Input: part model. Units: mm. Frame: model coordinates. A direction names the side the tool comes from. Round coordinates to 2 decimals unless told otherwise and drop trailing zeros. Loops run counter-clockwise (first coordinate to the right, second up) from the corner with the lowest first, then second, coordinate; pieces in that order, holes last. Notation, with made-up numbers: M 12,78.5 L 34,78.5 A26 cw 34,96.5 Z; hole C 69.5,42.25 d3. An arc over 180 degrees is marked long. Return JSON: item names as keys, results as strings. Group by question number.
1) Access query for faces 1 (the face through (40, -1, 10)), 2 (the face through (-115, 95, 20)), 3 (the face through (-1, 1, 20)), 4 (the face through (-40, -1, 10)). Directions: +Z, -Z, +X, -X, +Y, -Y. A direction counts if a zero-diameter tool reaches every point of the face in a straight line with its end or side. Return the directions, or none.
2) Contact query for flat-ended pins moving along their axis: P1, Ø8, axis at y = -4, z = 23.5, coming from the -X side; P2, Ø8, axis at x = 3.5, y = -25.5, coming from the +Z side; P3, Ø20, axis at x = -53.5, z = 19.5, coming from the -Y side. Output: stop coordinate, or through.
3) Section D-D (x = -71.5). Output: boundary loops of the cut face in (y, z), plus the area to 3 significant figures.
4) Section B-B (x = -32). Output: boundary loops of the cut face in (y, z), plus the area to 3 significant figures.
5) Section A-A (z = 7). Output: boundary loops of the cut face in (x, y), plus the area to 3 significant figures.
6) Material intervals for line 1 (X direction, y = 59.5, z = 17.5); line 2 (Y direction, x = 46, z = 26); line 3 (Z direction, x = -19.5, y = -14), sorted ascending. Write a range as from..to.
7) Section C-C (y = 44). Output: boundary loops of the cut face in (x, z), plus the area to 3 significant figures.
from build123d import *

# Parameters (mm, degrees)
SKETCH1_W           = 80
SKETCH1_H           = 160
BOSS_EXTRUDE1_DEPTH = 20
BOSS_EXTRUDE2_DEPTH = 40


with BuildPart() as part:
    # Sketch1 → Boss-Extrude1 (new body)
    with BuildSketch(Plane.XY):
        Rectangle(SKETCH1_W, SKETCH1_H)
    extrude(amount=BOSS_EXTRUDE1_DEPTH)

    # Sketch1<3> → Boss-Extrude2 (add)
    with BuildSketch(Plane.XY):
        Polygon((-115, 80), (-40, 80), (40, 80), (115, 80), (115, 110), (-115, 110), align=None)
    extrude(amount=BOSS_EXTRUDE2_DEPTH)


solid = part.part
Returned:
{
 "1": {"face 1": "+Z, -Z, +X, -Y", "face 2": "+Z, -Z, -X, +Y, -Y", "face 3": "+Z, +X, -X, -Y", "face 4": "+Z, -Z, -X, -Y"},
 "2": {"P1": "stops at x = -40", "P2": "stops at z = 20", "P3": "stops at y = 80"},
 "3": {"outline": "M 80,0 L 110,0 L 110,40 L 80,40 Z", "area": "1,200 mm^2"},
 "4": {"outline": "M -80,0 L 110,0 L 110,40 L 80,40 L 80,20 L -80,20 Z", "area": "4,400 mm^2"},
 "5": {"outline": "M -115,80 L -40,80 L -40,-80 L 40,-80 L 40,80 L 115,80 L 115,110 L -115,110 Z", "area": "19,700 mm^2"},
 "6": {"line 1": "x = -40..40", "line 2": "y = 80..110", "line 3": "z = 0..20"},
 "7": {"outline": "M -40,0 L 40,0 L 40,20 L -40,20 Z", "area": "1,600 mm^2"}
}
